Input: part model. Units: mm. Frame: model coordinates. Round coordinates to 2 decimals unless told otherwise and drop trailing zeros. Order: outer loops, then holes, each group sorted by start corner. A loop starts at its lowest first (then second) coordinate and runs counter-clockwise, first axis right, second up. Notation, with made-up numbers: (67, 58) -> (119, 58) arc R22 ccw to (119, 88) -> close; hole circle Ø9 at (23.25, 59). An arc over 180 degrees is marked (long way). Use a Markdown table: item, result.
from build123d import *

# Parameters (mm, degrees)
BOSS_EXTRUDE1_DEPTH = 6.35
SKETCH2_R           = 3.3655
CUT_EXTRUDE1_DEPTH  = 7.35


with BuildPart() as part:
    # Sketch1 → Boss-Extrude1 (new body)
    with BuildSketch(Plane(origin=(0, 0, 0), x_dir=(1, 0, 0), z_dir=(0, 1, 0))):
        Polygon((0, 0), (0, 327.025), (279.580480146, 72.886286408), align=None)
    extrude(amount=BOSS_EXTRUDE1_DEPTH)

    # Sketch2 → Cut-Extrude1 (cut, through all)
    with BuildSketch(Plane(origin=(0, 6.35, 0), x_dir=(1, 0, 0), z_dir=(0, 1, 0))):
        with Locations((9.525, 25.4)):
            Circle(SKETCH2_R)
        with Locations((9.525, 165.1)):
            Circle(SKETCH2_R)
        with Locations((9.525, 304.8)):
            Circle(SKETCH2_R)
        with Locations((22.175659142, 15.624524524)):
            Circle(SKETCH2_R)
        with Locations((132.778926013, 44.458659806)):
            Circle(SKETCH2_R)
        with Locations((243.382192884, 73.292795089)):
            Circle(SKETCH2_R)
    extrude(amount=-CUT_EXTRUDE1_DEPTH, mode=Mode.SUBTRACT)


solid = part.part
1) Pin query (flat end, axial travel): pin 1 Ø1 at (x, y) = (63.5, 5) entering from -Z; pin 2 Ø2 at (x, y) = (162, 4.5) entering from +Z; pin 3 Ø2 at (x, y) = (67, 2.5) entering from +Z. Return the tip coordinate at first contact, or that it passes through.
Results found:
| item | result |
|---|---|
| pin 1 | stops at z = -269.76 |
| pin 2 | stops at z = -41.97 |
| pin 3 | stops at z = -17.21 |
2) Cut plane C-C on x = 143. Return loops of the section in (y, z), and give its area (3 significant figures).
Results found:
| item | result |
|---|---|
| outline | (0, -197.04) -> (6.35, -197.04) -> (6.35, -37.28) -> (0, -37.28) -> close |
| area | 1,010 mm² |
3) Line query: L1, parallel to X at y = 2.25, z = -307.5; L2, parallel to X at y = 4.25, z = -165.1; L3, parallel to X at y = 3.5, z = -147.5. Output: solid intervals per line, ascending. Write a range as [from, to].
Results found:
| item | result |
|---|---|
| L1 | x = [0, 7.52], [11.53, 21.48] |
| L2 | x = [0, 6.16], [12.89, 178.14] |
| L3 | x = [0, 197.5] |
4) Pull-direction query (X, two-part tool) for faces 1 (the flat face through (137.833, 3.131, -201.735)), 2 (the flat face through (80, 0, -129)), 3 (the cylindrical face through (19.695, 3.219, -17.899)); classes: +X half, -X half, draft (parallel to the pull), parting line (faces both ways), or undercut.
Results found:
| item | result |
|---|---|
| face 1 | +X half |
| face 2 | draft |
| face 3 | undercut |
5) Cut plane B-B on z = -288. Return loops of the section in (x, y), and give its area (3 significant figures).
Results found:
| item | result |
|---|---|
| outline | (0, 0) -> (42.93, 0) -> (42.93, 6.35) -> (0, 6.35) -> close |
| area | 273 mm² |
6) Cut plane A-A on y = 3.25. Return loops of the section in (x, z) (1 decimal), and give its area (3 significant figures).
Results found:
| item | result |
|---|---|
| outline | (0, -327) -> (279.6, -72.9) -> (0, 0) -> close; hole circle Ø6.7 at (9.5, -304.8); hole circle Ø6.7 at (9.5, -165.1); hole circle Ø6.7 at (9.5, -25.4); hole circle Ø6.7 at (22.2, -15.6); hole circle Ø6.7 at (132.8, -44.5); hole circle Ø6.7 at (243.4, -73.3) |
| area | 45,500 mm² |
